The model under review builds one solid part; all positions refer to its coordinate system, in mm. Face numbers are marked on the shaded views. Give positions to 0.01 mm unless a question says otherwise; leave off trailing zeros. Write each loop counter-clockwise with the first axis right and the second up, starting at its lowest first coordinate (ties: lowest second). Pieces come first, ordered by that corner, then holes. Notation, with made-up numbers: (33, 5) - (68, 5) arc R30 cw to (68, 33) - close; hole circle Ø6 at (-24.75, 81.25). An arc over 180 degrees is marked (long way). Write item = value, one per line.
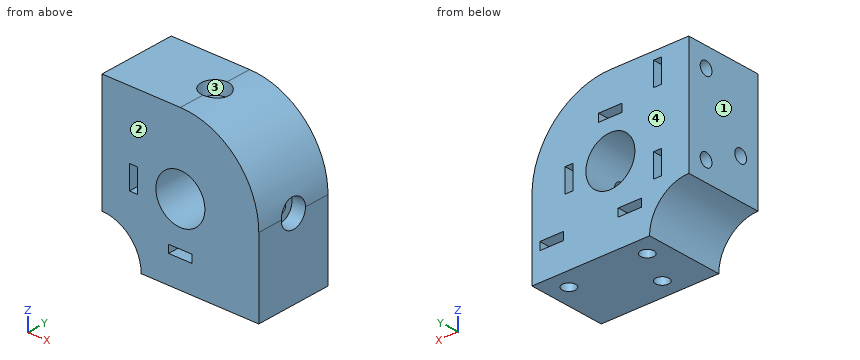
```python
from build123d import *

# Parameters (mm, degrees)
SKETCH1_W               = 40
SKETCH1_H               = 40
SKETCH1_R               = 6.25
BOSS_EXTRUDE1_DEPTH     = 20
SKETCH2_R               = 1.7
CUT_EXTRUDE1_DEPTH      = 11
CUT_EXTRUDE2_START      = -7
CUT_EXTRUDE2_DEPTH      = 2
CUT_EXTRUDE3_REACH      = 50.99
CUT_EXTRUDE3_END_RADIUS = 6.25
SKETCH4_R               = 1.7
CUT_EXTRUDE4_START      = -8.45
CUT_EXTRUDE4_DEPTH      = 2
SKETCH6_R               = 3.5
CUT_EXTRUDE5_DEPTH      = 3.45
FILLET1_R               = 20
CUT_EXTRUDE6_DEPTH      = 35.641016325


with BuildPart() as part:
    # Sketch1 → Boss-Extrude1 (new body)
    with BuildSketch(Plane(origin=(0, 0, 0), x_dir=(1, 0, 0), z_dir=(0, 1, 0))):
        Rectangle(SKETCH1_W, SKETCH1_H)
        with Locations(Location((0, 0, 0), (0, 0, 270))):
            Circle(SKETCH1_R, mode=Mode.SUBTRACT)
    extrude(amount=BOSS_EXTRUDE1_DEPTH)

    # Sketch2 → Cut-Extrude1 (cut)
    with BuildSketch(Plane.ZY.offset(20)):
        with Locations((-5, 15)):
            Circle(SKETCH2_R)
        with Locations((15, 15)):
            Circle(SKETCH2_R)
        with Locations((0, 5)):
            Circle(SKETCH2_R)
    cut_extrude1 = extrude(amount=-CUT_EXTRUDE1_DEPTH, mode=Mode.SUBTRACT)

    # Sketch3 → Cut-Extrude2 (cut)
    with BuildSketch(Plane.ZY.offset(20).offset(CUT_EXTRUDE2_START)):
        Polygon((-8, 12), (-2, 12), (-2, 18), (-2, 20), (-8, 20), (-8, 18), align=None)
        Polygon((12, 12), (18, 12), (18, 18), (18, 20), (12, 20), (12, 18), align=None)
        Polygon((-3, 8), (3, 8), (3, 2), (3, 0), (-3, 0), (-3, 2), align=None)
    cut_extrude2 = extrude(amount=-CUT_EXTRUDE2_DEPTH, mode=Mode.SUBTRACT)

    # Cut-Extrude3: up to this cylinder (the profile starts outside it)
    cut_extrude3_end = Plane(origin=(0, 10, 0), z_dir=(0, -1, 0)) * Cylinder(CUT_EXTRUDE3_END_RADIUS, 115.48, mode=Mode.PRIVATE)
    # Sketch4 → Cut-Extrude3 (cut, up to the surface)
    with BuildSketch(Plane.XY.offset(20), mode=Mode.PRIVATE) as cut_extrude3_sk1:
        with Locations((0, 10)):
            Circle(SKETCH4_R)
    cut_extrude3_tool1 = extrude(cut_extrude3_sk1.sketch, amount=-CUT_EXTRUDE3_REACH, mode=Mode.PRIVATE) - cut_extrude3_end
    cut_extrude3 = cut_extrude3_tool1.solids().sort_by_distance((0, 10, 20))[0]
    add(cut_extrude3, mode=Mode.SUBTRACT)

    # Sketch5 → Cut-Extrude4 (cut)
    with BuildSketch(Plane.XY.offset(20).offset(CUT_EXTRUDE4_START)):
        Polygon((-3, 13), (-3, 20), (3, 20), (3, 13), (3, 7), (-3, 7), align=None)
    cut_extrude4 = extrude(amount=-CUT_EXTRUDE4_DEPTH, mode=Mode.SUBTRACT)

    # Sketch6 → Cut-Extrude5 (cut)
    with BuildSketch(Plane.XY.offset(20)):
        with Locations((0, 10)):
            Circle(SKETCH6_R)
    cut_extrude5 = extrude(amount=-CUT_EXTRUDE5_DEPTH, mode=Mode.SUBTRACT)

    # Mirror1: Cut-Extrude1, Cut-Extrude2, Cut-Extrude3, Cut-Extrude4, Cut-Extrude5 across plane
    add(cut_extrude1.mirror(Plane(origin=(0, 0, 0), x_dir=(0.7071067811865476, 0, 0.7071067811865476), z_dir=(-0.7071067811865477, 0, 0.7071067811865475))), mode=Mode.SUBTRACT)
    add(cut_extrude2.mirror(Plane(origin=(0, 0, 0), x_dir=(0.7071067811865476, 0, 0.7071067811865476), z_dir=(-0.7071067811865477, 0, 0.7071067811865475))), mode=Mode.SUBTRACT)
    add(cut_extrude3.mirror(Plane(origin=(0, 0, 0), x_dir=(0.7071067811865476, 0, 0.7071067811865476), z_dir=(-0.7071067811865477, 0, 0.7071067811865475))), mode=Mode.SUBTRACT)
    add(cut_extrude4.mirror(Plane(origin=(0, 0, 0), x_dir=(0.7071067811865476, 0, 0.7071067811865476), z_dir=(-0.7071067811865477, 0, 0.7071067811865475))), mode=Mode.SUBTRACT)
    add(cut_extrude5.mirror(Plane(origin=(0, 0, 0), x_dir=(0.7071067811865476, 0, 0.7071067811865476), z_dir=(-0.7071067811865477, 0, 0.7071067811865475))), mode=Mode.SUBTRACT)

    # Fillet1
    # the kernel refuses this fillet: 20 mm, written as the material it takes off along each edge
    with BuildSketch(Plane(origin=(20, -50, 20), x_dir=(-1, 0, 0), z_dir=(0, 1, 0))) as fillet1_piece_1:
        with BuildLine():
            CenterArc((FILLET1_R, -FILLET1_R), FILLET1_R, 90, 90)
            Line((0, -FILLET1_R), (0, 0))
            Line((0, 0), (FILLET1_R, 0))
        make_face()
    extrude(amount=120, mode=Mode.SUBTRACT)

    # Sketch7 → Cut-Extrude6 (cut, through all)
    with BuildSketch(Plane(origin=(0, 20, 0), x_dir=(1, 0, 0), z_dir=(0, 1, 0))):
        with BuildLine():
            Line((-20, 10), (-20, 20))
            Line((-20, 20), (-10, 20))
            ThreePointArc((-10, 20), (-12.928932188, 12.928932188), (-20, 10))
        make_face()
    extrude(amount=-CUT_EXTRUDE6_DEPTH, mode=Mode.SUBTRACT)


solid = part.part
```
1. Take a section at D-D on x = -14.5. Give the boundary of the cut face in (y, z).
Findings below:
outline = (0, -11.65) - (20, -11.65) - (20, 20) - (0, 20) - close; hole circle Ø3.4 at (5, 0); hole circle Ø3.4 at (15, -5); hole circle Ø3.4 at (15, 15)
2. Insertion check: P1, Ø4, axis at y = 15, z = 15, coming from the +X side; P2, Ø1, axis at x = -0.5, y = 5.5, coming from the -Z side; P3, Ø1.6, axis at y = 12, z = 10.5, coming from the +X side. Each pin has a flat end and moves straight along its axis. Give the tip position at first contact, or say it passes through.
Findings below:
P1 = 15.2
P2 = -9
P3 = 17.49
3. Take a section at A-A on y = 17.75. Count the separate pieces of the cut face and the enclosed holes in it, and give its area (3 significant figures).
Findings below:
separate_pieces = 1
enclosed_holes = 7
area = 1,240 mm²
4. Draft analysis for pull direction Y (two halves, no side actions). For the marked faces 1, 2, 3 and 4, state which applies: +Y half, -Y half, draft (parallel to the pull), parting line (faces both ways), or undercut.
Findings below:
face_1 = draft
face_2 = -Y half
face_3 = undercut
face_4 = +Y half
5. Take a section at B-B on z = 15. Give the boundary of the cut face in (x, y).
Findings below:
outline = (-20, 0) - (13.23, 0) - (13.23, 20) - (-11, 20) - (-11, 16.7) - (-9, 16.7) - (-9, 13.3) - (-11, 13.3) - (-11, 12) - (-13, 12) - (-13, 13.3) - (-20, 13.3) - close; (-20, 16.7) - (-13, 16.7) - (-13, 20) - (-20, 20) - close; hole circle Ø3.4 at (0, 10)
6. Take a section at C-C on z = 4. Give the boundary of the cut face in (x, y).
Findings below:
outline = (-20, 0) - (-4.8, 0) - (-4.8, 20) - (-20, 20) - close; (4.8, 0) - (19.6, 0) - (19.6, 20) - (4.8, 20) - close
7. For line 1 (Y direction, x = 0, z = 8.65); line 2 (Y direction, x = 0, z = 17); line 3 (Z direction, x = -12.5, y = 12.25), list the stretches that pass through material, from the lowest coordinate up. Write a range as from..to.
Findings below:
line_1 = 0..8.3, 11.7..20
line_2 = 0..6.5, 13.5..20
line_3 = -13.39..-8, -2..12, 18..20
